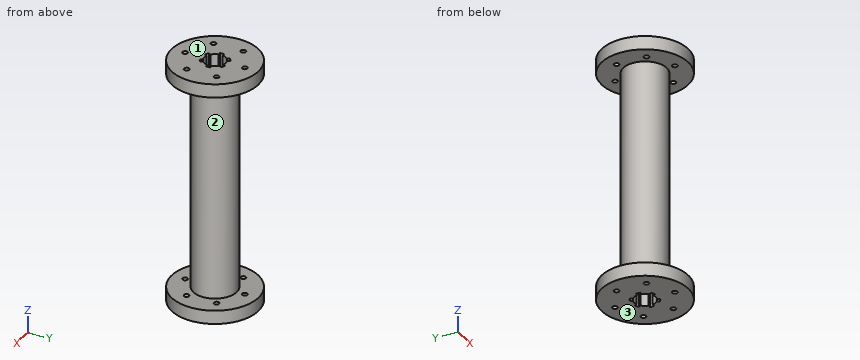
Autodesk Inventor part; units mm, degrees
ref_plane "YZ Plane" through (0, 0, 0) normal (1, 0, 0) x (0, 1, 0)
ref_plane "XZ Plane" through (0, 0, 0) normal (0, 1, 0) x (-1, 0, 0)
ref_plane "XY Plane" through (0, 0, 0) normal (0, 0, 1) x (1, 0, 0)
sketch "草图1" plane through (0, 0, 0) normal (0, 0, 1) x (1, 0, 0)
  circle A0 centre (0, 0) radius 80
  dimension "d0" = 160
extrude "拉伸1" add sketch "草图1" along normal blind 25
sketch "草图2" plane through (0, 0, 25) normal (0, 0, 1) x (1, 0, 0)
  circle A0 centre (0, 0) radius 40
  dimension "d3" = 80
extrude "拉伸2" add sketch "草图2" along normal blind 400
sketch "草图3" plane through (0, 0, 0) normal (0, 0, -1) x (-1, 0, 0)
  circle A0 centre (0, 55) radius 4.7538
  line L0 (0, 0) -> (0, 9.1463)
  dimension "d6" = 9.1463
  dimension "d7" = 55
extrude "拉伸3" cut sketch "草图3" against normal through all
pattern_circular "环形阵列1" count 6 over 360 about axis through (0, 0, -10) along (0, 0, 1) of "拉伸3"
pattern_linear "矩形阵列1" count 2 spacing 425 along (0, 0, 1) of "拉伸3", "环形阵列1", "拉伸1"
sketch "草图4" plane through (0, 0, 0) normal (0, 0, -1) x (-1, 0, 0)
  circle A0 centre (0, 0) radius 20
  dimension "d16" = 40
extrude "拉伸4" cut sketch "草图4" against normal through all
sketch "草图5" plane through (0, 0, 0) normal (0, 0, -1) x (-1, 0, 0)
  circle A0 centre (0, 0) radius 25
  circle A1 centre (0, 0) radius 20
  circle A2 centre (0, 0) radius 20
  line L0 (24.6779, 4) -> (19.5959, 4)
  line L1 (24.6779, -4) -> (19.5959, -4)
  line L2 (0, 0) -> (7.5201, 0)
  dimension "d19" = 50
  dimension "d20" = 7.5201
  dimension "d21" = 4
  dimension "d22" = 8
extrude "拉伸5" cut sketch "草图5" against normal through all contours A0 L1 A1 L0 picked at (21.5439, 2.2304)
pattern_circular "环形阵列2" count 6 over 360 about axis through (0, 0, -10) along (0, 0, 1) of "拉伸5"
properties part number "主动轮连接筒"
Design review of the part built by this model. Coordinates are the model's own, in mm. Face numbers are marked on the shaded views. Round coordinates to 2 decimals unless told otherwise and drop trailing zeros. Loops run counter-clockwise (first coordinate to the right, second up) from the corner with the lowest first, then second, coordinate; pieces in that order, holes last. Notation, with made-up numbers: (83, 11) - (93, 11) arc R28 cw to (93, 48) - close; hole circle Ø6 at (73, 29.25). An arc over 180 degrees is marked (long way). One line per item, written item: value. Start each with the question number.
1) Insertion check: pin 1 Ø5.5 at (x, y) = (0, 55) entering from +Z; pin 2 Ø4 at (x, z) = (-21.5, 282.5) entering from +Y; pin 3 Ø5 at (x, z) = (6.5, 211) entering from +Y; pin 4 Ø2 at (y, z) = (-4.5, 108) entering from -X. Each pin has a flat end and moves straight along its axis. Give the tip position at first contact, or say it passes through.
2) Draft analysis for pull direction Z (two halves, no side actions). For the marked faces 1, 2 and 3, state which applies: +Z half, -Z half, draft (parallel to the pull), parting line (faces both ways), or undercut.
3) Consider section C-C on z = 138. Give the boundary of the cut face in (x, y).
4) Consider section A-A on y = 55. Give the boundary of the cut face in (x, z).
5) Consider section D-D on y = -65. Give the boundary of the cut face in (x, z).
6) To check wall thickness, follow L1, parallel to Y at x = -15, z = 373; L2, parallel to Y at x = 14.5, z = 279; L3, parallel to Z at x = -23, y = -52. State the ranges of each line that lie inside material, in increasing order. Write a range as from..to.
7) Consider section B-B on x = -62. Give the boundary of the cut face in (y, z), then the cut area to 3 significant figures.
Reported:
1. pin 1: passes through
1. pin 2: stops at y = 34.92
1. pin 3: stops at y = 39.8
1. pin 4: stops at x = -39.85
2. face 1: +Z half
2. face 2: undercut
2. face 3: -Z half
3. outline: circle Ø80 at (0, 0); hole (-24.68, -4) - (-19.6, -4) arc R20 ccw to (-13.26, -14.97) - (-15.8, -19.37) arc R25 ccw to (-8.87, -23.37) - (-6.33, -18.97) arc R20 ccw to (6.33, -18.97) - (8.87, -23.37) arc R25 ccw to (15.8, -19.37) - (13.26, -14.97) arc R20 ccw to (19.6, -4) - (24.68, -4) arc R25 ccw to (24.68, 4) - (19.6, 4) arc R20 ccw to (13.26, 14.97) - (15.8, 19.37) arc R25 ccw to (8.87, 23.37) - (6.33, 18.97) arc R20 ccw to (-6.33, 18.97) - (-8.87, 23.37) arc R25 ccw to (-15.8, 19.37) - (-13.26, 14.97) arc R20 ccw to (-19.6, 4) - (-24.68, 4) arc R25 ccw to start
4. outline: (-58.09, 0) - (-4.75, 0) - (-4.75, 25) - (-58.09, 25) - close; (-58.09, 425) - (-4.75, 425) - (-4.75, 450) - (-58.09, 450) - close; (4.75, 0) - (58.09, 0) - (58.09, 25) - (4.75, 25) - close; (4.75, 425) - (58.09, 425) - (58.09, 450) - (4.75, 450) - close
5. outline: (-46.64, 0) - (46.64, 0) - (46.64, 25) - (-46.64, 25) - close; (-46.64, 425) - (46.64, 425) - (46.64, 450) - (-46.64, 450) - close
6. L1: y = -37.08..-20, -17.98..-13.23, 13.23..17.98, 20..37.08
6. L2: y = -37.28..-20.37, -17.11..-13.77, 13.77..17.11, 20.37..37.28
6. L3: z = 0..25, 425..450
7. outline: (-50.56, 0) - (50.56, 0) - (50.56, 25) - (-50.56, 25) - close; (-50.56, 425) - (50.56, 425) - (50.56, 450) - (-50.56, 450) - close
7. area: 5,060 mm^2
